Part model, mm, in its own coordinate system. Face numbers are marked on the shaded views. A direction names the side the tool comes from. Coordinates: 2 decimals unless noted, no trailing zeros. Order: outer loops, then holes, each group sorted by start corner. A loop starts at its lowest first (then second) coordinate and runs counter-clockwise, first axis right, second up. Notation, with made-up numbers: M 88.25,87.25 L 112.25,87.25 A22 cw 112.25,104.25 Z; hole C -13,23 d6. An arc over 180 degrees is marked long. Answer in a Markdown table with one row per item. Add a question column.
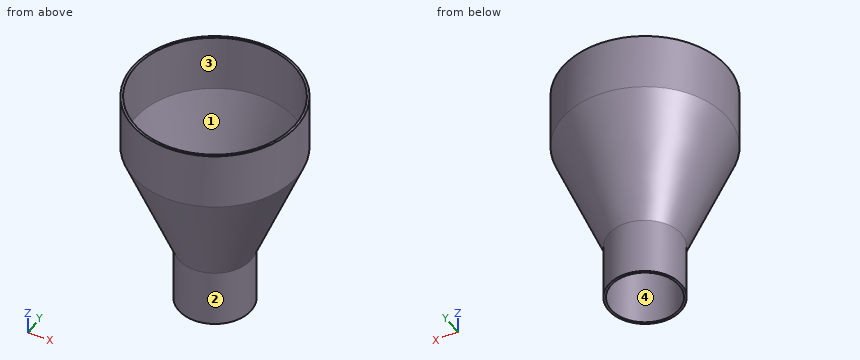
from build123d import *


# Not quite as in the source:
# - ends of sketch curves that miss each other by under 0.0002 mm in the source are joined


with BuildPart() as f1:
    # F0 (on Front) → F1 (revolve)
    with BuildSketch(Plane.XZ):
        Polygon((-15.113, -75.5039413649), (-15.113, -50.1039413649), (-16.1289999974, -50.1038177847), (-16.1289999982, -75.5039413649), align=None)
        Polygon((-15.1129998177, -50.1039412905), (-35.5600012367, -0.0001234082), (-36.5760016743, 7.015e-07), (-16.1290002526, -50.1038178889), align=None)
        Polygon((-36.5760016743, 7.015e-07), (-35.5600012367, -0.0001228868), (-35.56, 25.3998765918), (-36.5759999982, 25.3998765918), align=None)
    revolve(axis=Axis((0, 0, -37.7519706824), (0, 0, -1)))


solid = f1.part
(1) Wall check: line 1 (Y direction, x = 0, z = 19); line 2 (Y direction, x = 0, z = -57); line 3 (X direction, y = -9.5, z = -71). Give the ranges that are in metal, low to high.
(2) 3-axis set-ups, long thin cutter, end or side, ignore diameter. For the marked faces 3 and 4: which of +Z, -Z, +X, -X, +Y, -Y reach the whole face in a straight line?
(3) Drop flat-ended pins along their axis: P1, Ø1, axis at x = -3.5, z = -3.5, coming from the -Y side; P2, Ø8, axis at x = 13, y = -20, coming from the +Z side; P3, Ø8, axis at x = 26, y = -11, coming from the -Z side. Give the stop position or say it passes through.
(4) Slice it at D-D (z = -45). List the corners of the cut face in (x, y), and give its area (3 significant figures).
(5) Slice it at C-C (z = 5.5). List the corners of the cut face in (x, y), and give its area (3 significant figures).
(6) Pull direction Y, two halves, no side cores. Call the marked faces 1 and 2: pulls with the +Y half, pulls with the -Y half, needs draft (parallel to the pull), parting line crosses it, or undercut.
(7) Slice it at A-A (x = 0). List the corners of the cut face in (y, z).
Computed:
| question | item | result |
|---|---|---|
| 1 | line 1 | y = -36.58 to -35.56, 35.56 to 36.58 |
| 1 | line 2 | y = -16.13 to -15.11, 15.11 to 16.13 |
| 1 | line 3 | x = -13.03 to -11.75, 11.75 to 13.03 |
| 2 | face 3 | +Z |
| 2 | face 4 | +Z, -Z |
| 3 | P1 | stops at y = -35.18 |
| 3 | P2 | stops at z = -18.88 |
| 3 | P3 | stops at z = -30.25 |
| 4 | outline | C 0,0 d36.42; hole C 0,0 d34.39 |
| 4 | area | 113 mm^2 |
| 5 | outline | C 0,0 d73.15; hole C 0,0 d71.12 |
| 5 | area | 230 mm^2 |
| 6 | face 1 | undercut |
| 6 | face 2 | parting line crosses it |
| 7 | outline | M -36.58,0 L -16.13,-50.1 L -16.13,-75.5 L -15.11,-75.5 L -15.11,-50.1 L -35.56,0 L -35.56,25.4 L -36.58,25.4 Z; M 15.11,-75.5 L 16.13,-75.5 L 16.13,-50.1 L 36.58,0 L 36.58,25.4 L 35.56,25.4 L 35.56,0 L 15.11,-50.1 Z |
